Work out the finished part from the listing and answer in its coordinate system (mm). A direction names the side the tool comes from. Coordinates: 2 decimals unless noted, no trailing zeros. Write each loop counter-clockwise with the first axis right and the second up, starting at its lowest first coordinate (ties: lowest second). Pieces come first, ordered by that corner, then holes. Notation, with made-up numbers: (-18.75, 0.25) - (1.25, 0.25) arc R23 ccw to (1.25, 38.25) - close; hole circle Ø10 at (-4.75, 58.25). An arc over 180 degrees is marked (long way). Use one line per item in the form item = value. Start each with the question number.
Item 1: A cutting plane is placed at D-D (z = 1). Write down the section's boundary in (x, y), then the cut area to 3 significant figures.
Item 2: For faces 1 (the flat face through (-30.5, 2, 14)), 2 (the flat face through (4.762, 2, 0)), 3 (the flat face through (23.5, 2, 26)), determine the directions among +Z, -Z, +X, -X, +Y, -Y from which every point of the face is accessible in a straight line to the end or side of a thin tool.
Item 3: Consider probe 1 along X at (y, z) = (1.85, 24); probe 2 along X at (y, z) = (2.9, 15) (3 decimals); probe 3 along X at (y, z) = (2.95, 3.5). Determine where each line is inside the solid, lowest interval first.
Item 4: A cutting plane is placed at B-B (z = 15). Write down the section's boundary in (x, y) (1 decimal), then the cut area to 3 significant figures.
Item 5: A cutting plane is placed at A-A (x = 12). Write down the section's boundary in (y, z).
Item 6: A cutting plane is placed at C-C (y = 1.7). Give the number of separate pieces and of enclosed holes in the cut face, then the cut area to 3 significant figures.
Item 7: Determine the mould class of faces 4 (the flat face through (0, 2, 23.238)), 5 (the flat face through (23.641, 2.348, -10.553)), 6 (the cylindrical face through (-16.72, 2.35, -18.61)), 7 (the flat face through (27, 2, 28)) for opening direction X: released by +X, released by -X, zero draft, split by the parting line, or undercut.
Item 8: Given pin 1 (1.4 mm diameter, centred on x = 8.5, y = 3, fed in from +Z); pin 2 (1.4 mm diameter, centred on y = 2.5, z = -1, fed in from -X); pin 3 (1.5 mm diameter, centred on x = -24.5, y = 1, fed in from -Z), each flat-ended and moving along its own axis, determine where each tip first touches the part or whether it passes through.
from build123d import *

# Parameters (mm, degrees)
SKETCH1_R           = 1.625
SKETCH1_R_2         = 2.375
SKETCH1_R_3         = 3
BOSS_EXTRUDE1_DEPTH = 4.7625
SKETCH2_R           = 0.5
CUT_EXTRUDE1_DEPTH  = 5.7625


with BuildPart() as part:
    # Sketch1 → Boss-Extrude1 (new body)
    with BuildSketch(Plane(origin=(0, 0, 0), x_dir=(1, 0, 0), z_dir=(0, 1, 0))):
        with BuildLine():
            Line((-4.7625, -4.200130206), (-4.7625, 4.200130206))
            ThreePointArc((-4.7625, 4.200130206), (-2.612630206, 5.787630206), (0, 6.35))
            Line((0, 6.35), (0, 19))
            Line((0, 19), (-15, 19))
            ThreePointArc((-15, 19), (-16.738947924, 18.602229881), (-18.132045087, 17.488030058))
            Line((-18.132045087, 17.488030058), (-29.306561995, 3.42104133))
            ThreePointArc((-29.306561995, 3.42104133), (-30.193076688, 1.811616547), (-30.5, 0))
            Line((-30.5, 0), (-30.5, -28))
            Line((-30.5, -28), (-23.5, -28))
            Line((-23.5, -28), (-23.5, -23.2375))
            Line((-23.5, -23.2375), (0, -23.2375))
            Line((0, -23.2375), (0, -6.35))
            ThreePointArc((0, -6.35), (-2.612630206, -5.787630206), (-4.7625, -4.200130206))
        make_face()
        with Locations((-15, 15)):
            Circle(SKETCH1_R, mode=Mode.SUBTRACT)
        with Locations((-15, -15)):
            Circle(SKETCH1_R, mode=Mode.SUBTRACT)
        with Locations((-25, 0)):
            Circle(SKETCH1_R_2, mode=Mode.SUBTRACT)
        with Locations((-12, -6)):
            Circle(SKETCH1_R_3, mode=Mode.SUBTRACT)
        with Locations((-12, 6)):
            Circle(SKETCH1_R_3, mode=Mode.SUBTRACT)
    boss_extrude1 = extrude(amount=BOSS_EXTRUDE1_DEPTH)

    # Mirror1: Boss-Extrude1 across plane
    add(boss_extrude1.mirror(Plane(origin=(0, 4.7625, 6.35), x_dir=(0, 0, 1), z_dir=(-1, 0, 0))))

    # Sketch2 → Cut-Extrude1 (cut, through all)
    with BuildSketch(Plane(origin=(0, 4.7625, 0), x_dir=(1, 0, 0), z_dir=(0, 1, 0))):
        with Locations((-23.25, -23.4875)):
            Circle(SKETCH2_R)
        with Locations((23.25, -23.4875)):
            Circle(SKETCH2_R)
    extrude(amount=-CUT_EXTRUDE1_DEPTH, mode=Mode.SUBTRACT)


solid = part.part
Answer:
q1.outline = (-30.5, 0) - (-27.15, 0) - (-27.15, 4.76) - (-30.5, 4.76) - close; (-22.85, 0) - (-4.76, 0) - (-4.76, 4.76) - (-22.85, 4.76) - close; (4.76, 0) - (22.85, 0) - (22.85, 4.76) - (4.76, 4.76) - close; (27.15, 0) - (30.5, 0) - (30.5, 4.76) - (27.15, 4.76) - close
q1.area = 204 mm²
q2.face_1 = +Z, -Z, -X, +Y, -Y
q2.face_2 = +Y, -Y
q2.face_3 = +Z, +Y, -Y
q3.probe_1 = -30.5 to -23.5, 23.5 to 30.5
q3.probe_2 = -30.5 to -16.625, -13.375 to 13.375, 16.625 to 30.5
q3.probe_3 = -30.5 to -13.66, -10.34 to -4.76, 4.76 to 10.34, 13.66 to 30.5
q4.outline = (-30.5, 0) - (-16.6, 0) - (-16.6, 4.8) - (-30.5, 4.8) - close; (-13.4, 0) - (13.4, 0) - (13.4, 4.8) - (-13.4, 4.8) - close; (16.6, 0) - (30.5, 0) - (30.5, 4.8) - (16.6, 4.8) - close
q4.area = 260 mm²
q5.outline = (0, -19) - (4.76, -19) - (4.76, -9) - (0, -9) - close; (0, -3) - (4.76, -3) - (4.76, 3) - (0, 3) - close; (0, 9) - (4.76, 9) - (4.76, 23.24) - (0, 23.24) - close
q6.separate_pieces = 1
q6.enclosed_holes = 11
q6.area = 2,120 mm²
q7.face_4 = undercut
q7.face_5 = released by +X
q7.face_6 = released by -X
q7.face_7 = zero draft
q8.pin_1 = 23.24
q8.pin_2 = -30.49
q8.pin_3 = -10.42
